Check sheet for the drawn part. Datum: minimum x, y, z corner. Units: mm. A direction names the side the tool comes from. Give positions to 0.01 mm unless a question says otherwise; leave off trailing zeros. Write each loop counter-clockwise with the first axis right and the second up, starting at its lowest first coordinate (ties: lowest second). Pieces come first, ordered by that corner, then holes. Notation, with made-up numbers: (20, 54.5) - (71, 54.5) arc R21 cw to (71, 62.5) - close; hole circle Ø11 at (-28, 33). An arc over 180 degrees is marked (long way). Return JSON: item names as keys, results as strings. Group by question number.
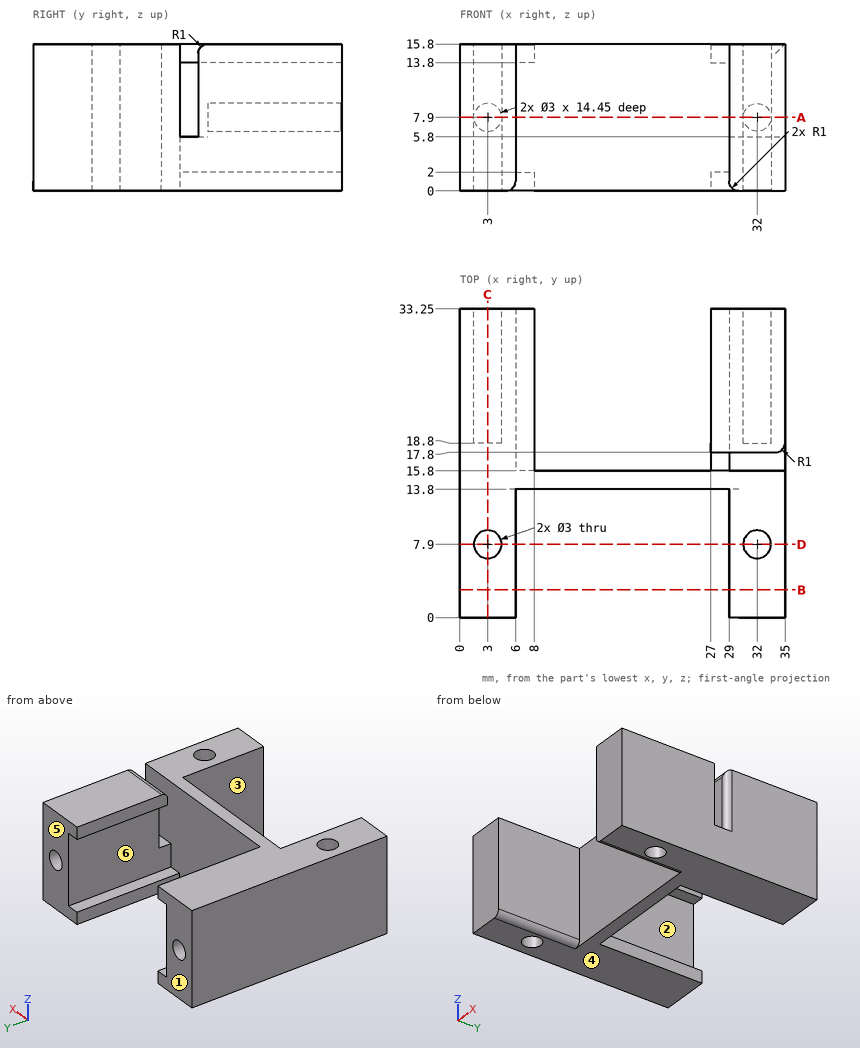
Item 1: Section check A-A on z = 7.9. Record the cut outline in (x, y).
Item 2: Section check B-B on y = 3. Record the cut outline in (x, z), plus the area to 3 significant figures.
Item 3: Mould release check, pull along Z, two halves, no side actions. Record for the marked faces 4, 5 and 6: +Z half, -Z half, draft (parallel to the pull), parting line (faces both ways), or undercut.
Item 4: Material ranges on line 1 along Y through (x, z) = (32, 10.25); line 2 along X through (y, z) = (25.5, 7.9); line 3 along X through (y, z) = (7, 3.5), recorded low to high. Write a range as from..to.
Item 5: Access from +Z, -Z, +X, -X, +Y, -Y to the whole of each face (thin tool, end or side, straight path). Record for the marked faces 1, 2 and 3.
Item 6: Depth check by flat-ended pin: pin 1 (1.5 mm diameter, centred on x = 31.5, y = 17.5, fed in from +Z). Enter the tip coordinate at first touch or a pass-through.
Item 7: Section check C-C on x = 3. Record the cut outline in (y, z).
Item 8: Section check D-D on y = 7.9. Record the cut outline in (x, z).
Reply:
{
 "1": {"outline": "(0, 0) - (6, 0) - (6, 13.8) - (29, 13.8) - (29, 0) - (35, 0) - (35, 15.8) - (6, 15.8) - (6, 33.25) - (4.5, 33.25) - (4.5, 18.8) - (1.5, 18.8) - (1.5, 33.25) - (0, 33.25) - close; (29, 17.8) - (34, 17.8) arc R1 ccw to (35, 18.8) - (35, 33.25) - (33.5, 33.25) - (33.5, 18.8) - (30.5, 18.8) - (30.5, 33.25) - (29, 33.25) - close; hole circle Ø3 at (3, 7.9); hole circle Ø3 at (32, 7.9)"},
 "2": {"outline": "(0, 0) - (5, 0) arc R1 ccw to (6, 1) - (6, 15.8) - (0, 15.8) - close; (29, 1) arc R1 ccw to (30, 0) - (35, 0) - (35, 15.8) - (29, 15.8) - close", "area": "189 mm²"},
 "3": {"face 4": "-Z half", "face 5": "draft", "face 6": "undercut"},
 "4": {"line 1": "0..6.4, 9.4..15.8, 17.8..33.25", "line 2": "0..1.5, 4.5..6, 29..30.5, 33.5..35", "line 3": "0..1.8, 4.2..6, 29..30.8, 33.2..35"},
 "5": {"face 1": "+Z, -Z, +X, -X, +Y", "face 2": "+Y", "face 3": "+Z, -Z, -Y"},
 "6": {"pin 1": "z = 15.64"},
 "7": {"outline": "(0, 0) - (6.4, 0) - (6.4, 15.8) - (0, 15.8) - close; (9.4, 0) - (33.25, 0) - (33.25, 6.4) - (18.8, 6.4) - (18.8, 9.4) - (33.25, 9.4) - (33.25, 15.8) - (9.4, 15.8) - close"},
 "8": {"outline": "(0, 0) - (1.5, 0) - (1.5, 15.8) - (0, 15.8) - close; (4.5, 0) - (5, 0) arc R1 ccw to (6, 1) - (6, 15.8) - (4.5, 15.8) - close; (29, 1) arc R1 ccw to (30, 0) - (30.5, 0) - (30.5, 15.8) - (29, 15.8) - close; (33.5, 0) - (35, 0) - (35, 15.8) - (33.5, 15.8) - close"}
}
